```python
from build123d import *

# Parameters (mm, degrees)
CHAMFER1_SIZE           = 0.5
SKETCH2_OUTSIDE_W       = 108.196
SKETCH2_OUTSIDE_H       = 108.196
CUT_EXTRUDE1_DEPTH      = 21
CUT_EXTRUDE2_DEPTH      = 72.056315694
CUT_EXTRUDE2_DEPTH_BACK = 72.056315694
SKETCH6_R               = 4
CUT_EXTRUDE3_DEPTH      = 72.056315694
CIRPATTERN1_COUNT       = 2
CIRPATTERN1_ANGLE       = 90


with BuildPart() as part:
    # Sketch1 → Revolve1 (revolve)
    with BuildSketch(Plane.XY, mode=Mode.PRIVATE) as revolve1_sk:
        Polygon((-43, 40), (0, 40), (0, 35), (23, 35), (23, 0), (-43, 0), align=None)
    revolve(revolve1_sk.sketch.rotate(Axis((-50.16, 0, 0), (1, 0, 0)), 90), axis=Axis((-50.16, 0, 0), (1, 0, 0)))

    # Chamfer1
    chamfer1_edges = [part.edges().sort_by_distance(p)[0] for p in [
        (23, 0, -35),
    ]]
    chamfer(chamfer1_edges, length=CHAMFER1_SIZE)

    # Sketch2 outside → Cut-Extrude1 (cut)
    with BuildSketch(Plane.ZY.offset(43)):
        Rectangle(SKETCH2_OUTSIDE_W, SKETCH2_OUTSIDE_H)
        with BuildLine():
            Line((38.578346676, -10.569350395), (23.599719808, -4.365))
            ThreePointArc((23.599719808, -4.365), (24, 0), (23.599719808, 4.365))
            Line((23.599719808, 4.365), (38.578346676, 10.569350395))
            ThreePointArc((38.578346676, 10.569350395), (40, 0), (38.578346676, -10.569350395))
        make_face(mode=Mode.SUBTRACT)
        with BuildLine():
            Line((-10.569350395, 38.578346676), (-4.365, 23.599719808))
            ThreePointArc((-4.365, 23.599719808), (0, 24), (4.365, 23.599719808))
            Line((4.365, 23.599719808), (10.569350395, 38.578346676))
            ThreePointArc((10.569350395, 38.578346676), (0, 40), (-10.569350395, 38.578346676))
        make_face(mode=Mode.SUBTRACT)
        with BuildLine():
            Line((-10.569350395, -38.578346676), (-4.365, -23.599719808))
            ThreePointArc((-4.365, -23.599719808), (0, -24), (4.365, -23.599719808))
            Line((4.365, -23.599719808), (10.569350395, -38.578346676))
            ThreePointArc((10.569350395, -38.578346676), (0, -40), (-10.569350395, -38.578346676))
        make_face(mode=Mode.SUBTRACT)
        with BuildLine():
            Line((-38.578346676, 10.569350395), (-23.599719808, 4.365))
            ThreePointArc((-23.599719808, 4.365), (-24, 0), (-23.599719808, -4.365))
            Line((-23.599719808, -4.365), (-38.578346676, -10.569350395))
            ThreePointArc((-38.578346676, -10.569350395), (-40, 0), (-38.578346676, 10.569350395))
        make_face(mode=Mode.SUBTRACT)
    extrude(amount=-CUT_EXTRUDE1_DEPTH, mode=Mode.SUBTRACT)

    # Sketch4 → Cut-Extrude2 (cut, two sides: drawn at the far end of the back side and taken through both)
    with BuildSketch(Plane.ZY.offset(-CUT_EXTRUDE2_DEPTH_BACK)):
        with BuildLine():
            Line((-15.3, -4), (-11.313708499, -4))
            ThreePointArc((-11.313708499, -4), (12, 0), (-11.313708499, 4))
            Line((-11.313708499, 4), (-15.3, 4))
            Line((-15.3, 4), (-15.3, -4))
        make_face()
    extrude(amount=CUT_EXTRUDE2_DEPTH + CUT_EXTRUDE2_DEPTH_BACK, mode=Mode.SUBTRACT)

    # Sketch6 → Cut-Extrude3 (cut, through all)
    with BuildSketch(Plane(origin=(0, 0, 0), x_dir=(1, 0, 0), z_dir=(0, 1, 0))):
        with Locations(Location((5, 0, 0), (0, 0, 270))):
            Circle(SKETCH6_R)
    cut_extrude3 = extrude(amount=-CUT_EXTRUDE3_DEPTH, mode=Mode.SUBTRACT)

    # CirPattern1: Cut-Extrude3 ×2 about axis
    cirpattern1_axis = Axis((0, 0, 0), (-1, 0, 0))
    for i in range(1, CIRPATTERN1_COUNT):
        add(cut_extrude3.rotate(cirpattern1_axis, i * CIRPATTERN1_ANGLE / (CIRPATTERN1_COUNT - 1)), mode=Mode.SUBTRACT)


solid = part.part
```
Geometry: final body of the model. Coordinates: model frame, mm. A direction names the side the tool comes from. Coordinates: 2 decimals unless noted, no trailing zeros. Order: outer loops, then holes, each group sorted by start corner. A loop starts at its lowest first (then second) coordinate and runs counter-clockwise, first axis right, second up. Notation, with made-up numbers: (75.5, 20) - (124.5, 20) arc R20 cw to (124.5, 25) - close; hole circle Ø10 at (45.25, 15). An arc over 180 degrees is marked (long way). Return JSON: item names as keys, results as strings. Group by question number.
1. Cut plane C-C (x = -24). Output: boundary loops of the cut face in (y, z) (3 decimals).
2. Set-up query: faces 1 (the face through (-32.65, 31.19, -7.51)), 2 (the face through (-33, 24, 0)), 3 (the face through (-32.65, 30.98, 7.42)). Return all of +Z, -Z, +X, -X, +Y, -Y with unobstructed straight access to the full face (end or side cutting, diameter ignored); none if empty.
3. Material intervals for line 1 along X through (y, z) = (0, 20.25); line 2 along X through (y, z) = (-29, 0); line 3 along X through (y, z) = (11, -20.5), sorted ascending. Write a range as [from, to].
4. Pin query (flat end, axial travel): pin 1 (2 mm diameter, centred on x = -16.5, y = -19, fed in from -Z); pin 2 (8 mm diameter, centred on y = -17, z = 2, fed in from -X); pin 3 (2 mm diameter, centred on x = 10.5, z = -14, fed in from -Y). Return the tip coordinate at first contact, or that it passes through.
5. Cut plane D-D (x = -5). Output: boundary loops of the cut face in (y, z), plus the area to 3 significant figures.
6. Cut plane B-B (y = 0). Output: boundary loops of the cut face in (x, z), plus the area to 3 significant figures.
7. Cut plane A-A (z = 0). Output: boundary loops of the cut face in (x, y).
8. Pull-direction query (Y, two-part tool) for faces 4 (the face through (-32.65, 7.42, 30.98)), 5 (the face through (0, 35.4, -0.2)), 6 (the face through (-32.65, -30.98, 7.42)); classes: pulls with the +Y half, pulls with the -Y half, needs draft (parallel to the pull), parting line crosses it, or undercut.
Resolved:
{
 "1": {"outline": "(-38.578, -10.569) - (-23.6, -4.365) arc R24 cw to (-23.6, 4.365) - (-38.578, 10.569) arc R40 ccw to start; (-10.569, -38.578) arc R40 ccw to (10.569, -38.578) - (4.365, -23.6) arc R24 cw to (-4.365, -23.6) - close; (-10.569, 38.578) - (-4.365, 23.6) arc R24 cw to (4.365, 23.6) - (10.569, 38.578) arc R40 ccw to start; (23.6, -4.365) - (38.578, -10.569) arc R40 ccw to (38.578, 10.569) - (23.6, 4.365) arc R24 cw to start"},
 "2": {"face 1": "-Z, -X", "face 2": "-X", "face 3": "+Z, -X"},
 "3": {"line 1": "x = [-22, 1], [9, 23]", "line 2": "x = [-43, 1], [9, 23]", "line 3": "x = [-22, 23]"},
 "4": {"pin 1": "stops at z = -35.72", "pin 2": "stops at x = -22", "pin 3": "stops at y = -32.5"},
 "5": {"outline": "circle Ø80 at (0, 0); hole (-4, -15.3) - (4, -15.3) - (4, -11.31) arc R12 ccw (long way) to (-4, -11.31) - close", "area": "4,550 mm²"},
 "6": {"outline": "(-43, -40) - (0, -40) - (0, -35) - (22.5, -35) - (23, -34.5) - (23, -15.3) - (-22, -15.3) - (-22, -24) - (-43, -24) - close; (-43, 24) - (-22, 24) - (-22, 12) - (1, 12) - (1, 35) - (0, 35) - (0, 40) - (-43, 40) - close; (9, 12) - (23, 12) - (23, 34.5) - (22.5, 35) - (9, 35) - close", "area": "2,630 mm²"},
 "7": {"outline": "(-43, -40) - (0, -40) - (0, -35) - (1, -35) - (1, -12) - (-22, -12) - (-22, -24) - (-43, -24) - close; (-43, 24) - (-22, 24) - (-22, 12) - (23, 12) - (23, 34.5) - (22.5, 35) - (0, 35) - (0, 40) - (-43, 40) - close; (9, -35) - (22.5, -35) - (23, -34.5) - (23, -12) - (9, -12) - close"},
 "8": {"face 4": "pulls with the +Y half", "face 5": "needs draft", "face 6": "undercut"}
}
